Source: CAD feature listing. Evaluate the final solid. Frame: model axes, mm. Face numbers are marked on the shaded views. Round coordinates to 2 decimals unless told otherwise and drop trailing zeros. Order: outer loops, then holes, each group sorted by start corner. A loop starts at its lowest first (then second) coordinate and runs counter-clockwise, first axis right, second up. Notation, with made-up numbers: (55.25, -0.5) -> (100.25, -0.5) arc R32 ccw to (100.25, 28.5) -> close; hole circle Ø4 at (-23, -19). An arc over 180 degrees is marked (long way). One line per item, written item: value. Start each with the question number.
1) Pin query (flat end, axial travel): P1, Ø1, axis at x = 20, y = 22, coming from the +Z side; P2, Ø4, axis at x = -12.5, z = 50.5, coming from the +Y side; P3, Ø6, axis at x = -32.5, z = 99, coming from the -Y side. Return the tip coordinate at first contact, or that it passes through.
2) Ray query, L1, parallel to Z at x = 23, y = -14; L2, parallel to X at y = -7.5, z = 101; L3, parallel to Y at x = -42, z = -123.5. Return the intervals inside material, ascending.
3) Section C-C (z = -75.5). Return the cut outline in (x, y), and give its area (3 significant figures).
4) Section A-A (y = 0). Return the cut outline in (x, z), and give its area (3 significant figures).
5) Mould query, pull axis X, two halves, no side actions, for the marked faces 1 and 2. Classes: pulls with the +X half, pulls with the -X half, needs draft (parallel to the pull), parting line crosses it, or undercut.
6) Section D-D (x = -38). Return the cut outline in (y, z).
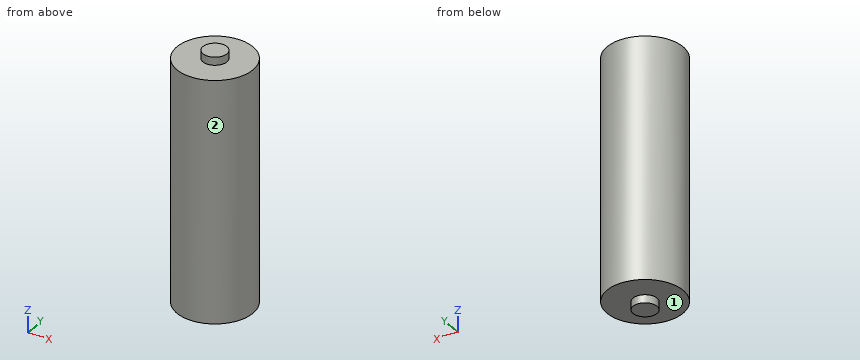
```python
from build123d import *

# Parameters (mm, degrees)
SKETCH1_R                = 47.5
BOSS_EXTRUDE1_DEPTH      = 150
BOSS_EXTRUDE2_DEPTH      = 10
BOSS_EXTRUDE2_DEPTH_BACK = 310
SKETCH2_R                = 15


with BuildPart() as part:
    # Sketch1 → Boss-Extrude1 (new, symmetric)
    with BuildSketch(Plane.XY):
        Circle(SKETCH1_R)
    extrude(amount=BOSS_EXTRUDE1_DEPTH, both=True)

    # Sketch2 → Boss-Extrude2 (add, two sides: drawn at the far end of the back side and taken through both)
    with BuildSketch(Plane.XY.offset(150).offset(-BOSS_EXTRUDE2_DEPTH_BACK)):
        Circle(SKETCH2_R)
    extrude(amount=BOSS_EXTRUDE2_DEPTH + BOSS_EXTRUDE2_DEPTH_BACK)


solid = part.part
```
Findings:
1. P1: z = 150
1. P2: y = 46.32
1. P3: y = -37.23
2. L1: -150 to 150
2. L2: -46.9 to 46.9
2. L3: -22.19 to 22.19
3. outline: circle Ø95 at (0, 0)
3. area: 7,090 mm2
4. outline: (-47.5, -150) -> (-15, -150) -> (-15, -160) -> (15, -160) -> (15, -150) -> (47.5, -150) -> (47.5, 150) -> (15, 150) -> (15, 160) -> (-15, 160) -> (-15, 150) -> (-47.5, 150) -> close
4. area: 29,100 mm2
5. face 1: needs draft
5. face 2: parting line crosses it
6. outline: (-28.5, -150) -> (28.5, -150) -> (28.5, 150) -> (-28.5, 150) -> close
